from build123d import *

# Parameters (mm, degrees)
F0_R     = 5
F1_DEPTH = 17.5514
F0_W     = 10
F0_H     = 25
F2_DEPTH = 20
F3_R     = 5
F4_DEPTH = 17.5514


with BuildPart() as f1:
    # F0 (on Right) → F1 (new body)
    with BuildSketch(Plane.YZ):
        Polygon((10, -20), (10, 20), (-10, 20), (-10, 5), (-10, -20), align=None)
        with Locations((0, -10)):
            Circle(F0_R, mode=Mode.SUBTRACT)
    extrude(amount=F1_DEPTH)

    # F0 (on Right) → F2 (join)
    with BuildSketch(Plane.YZ):
        with Locations((-15, -7.5)):
            Rectangle(F0_W, F0_H)
    extrude(amount=F2_DEPTH)

    # F3 (on face) → F4 (cut, through all)
    with BuildSketch(Plane.YZ):
        with Locations((0, 10)):
            Circle(F3_R)
    extrude(amount=F4_DEPTH, mode=Mode.SUBTRACT)


solid = f1.part
Here's how the part is built. I have some questions about the finished solid (model axes, mm). A direction names the side the tool comes from. Round coordinates to 2 decimals unless told otherwise and drop trailing zeros. Order: outer loops, then holes, each group sorted by start corner. A loop starts at its lowest first (then second) coordinate and runs counter-clockwise, first axis right, second up. Notation, with made-up numbers: (53, 22.5) -> (70, 22.5) arc R11 cw to (70, 32.5) -> close; hole circle Ø9 at (-21, 68). An arc over 180 degrees is marked (long way). Return JSON: item names as keys, results as strings.
Q1. If we section it at B-B on y = 0: List the corners of the cut face in (x, z) for me, plus the area to 3 significant figures.
Filled sheet:
{"outline": "(0, -20) -> (17.55, -20) -> (17.55, -15) -> (0, -15) -> close; (0, -5) -> (17.55, -5) -> (17.55, 5) -> (0, 5) -> close; (0, 15) -> (17.55, 15) -> (17.55, 20) -> (0, 20) -> close", "area": "351 mm^2"}
Q2. Which directions (+Z, -Z, +X, -X, +Y, -Y) give clear straight access to the entire face, cutting with the end or side of a thin tool? Please do faces 1 (the flat face through (10, -15, 5)), 2 (the flat face through (0, -5, 0)), 3 (the flat face through (19, -10, -8)).
Filled sheet:
{"face 1": "+Z, +X, -X, -Y", "face 2": "+Z, -Z, -X, +Y, -Y", "face 3": "+Z, -Z, +X, +Y"}
Q3. If we mould it in two halves opening along Z, with no side actions, what happens to faces 4 (the flat face through (10, -20, -8)), 5 (the flat face through (9, 0, 20)), 6 (the cylindrical face through (8.653, -0.651, -5.043))? For each: released by +Z, released by -Z, zero draft, split by the parting line, or undercut.
Filled sheet:
{"face 4": "zero draft", "face 5": "released by +Z", "face 6": "undercut"}
Q4. If we section it at D-D on z = 2: List the corners of the cut face in (x, y) for me.
Filled sheet:
{"outline": "(0, -20) -> (20, -20) -> (20, -10) -> (17.55, -10) -> (17.55, 10) -> (0, 10) -> close"}
Q5. I need wall thicknesses on line 1 along Z through (x, y) = (14, 0); line 2 along Y through (x, z) = (19.25, -4); line 3 along Y through (x, z) = (8.25, -9.5). Which ranges of each line are inside material? Lowest first, please. Write a range as from..to.
Filled sheet:
{"line 1": "z = -20..-15, -5..5, 15..20", "line 2": "y = -20..-10", "line 3": "y = -20..-4.97, 4.97..10"}
Q6. If we section it at C-C on z = 6: List the corners of the cut face in (x, y) for me.
Filled sheet:
{"outline": "(0, -10) -> (17.55, -10) -> (17.55, -3) -> (0, -3) -> close; (0, 3) -> (17.55, 3) -> (17.55, 10) -> (0, 10) -> close"}
Q7. For pin 1 Ø10 at (x, y) = (12, -16.5) entering from +Z; pin 2 Ø1.2 at (x, z) = (19, -12) entering from +Y; pin 3 Ø16 at (y, z) = (-0.5, -4) entering from +X; pin 4 Ø9 at (y, z) = (0, 10) entering from -X, each with a flat end and sliding along its axis, tell me the tip position at first contact or that it passes through.
Filled sheet:
{"pin 1": "stops at z = 5", "pin 2": "stops at y = -10", "pin 3": "stops at x = 17.55", "pin 4": "passes through"}
Q8. If we section it at A-A on z = 10: List the corners of the cut face in (x, y) for me.
Filled sheet:
{"outline": "(0, -10) -> (17.55, -10) -> (17.55, -5) -> (0, -5) -> close; (0, 5) -> (17.55, 5) -> (17.55, 10) -> (0, 10) -> close"}
